Source: CAD feature listing. Evaluate the final solid. Frame: model axes, mm. A direction names the side the tool comes from. Give positions to 0.01 mm unless a question says otherwise; leave off trailing zeros. Loops run counter-clockwise (first coordinate to the right, second up) from the corner with the lowest first, then second, coordinate; pieces in that order, holes last. Notation, with made-up numbers: (26.25, 43) -> (70.25, 43) arc R9 cw to (70.25, 55) -> close; hole circle Ø9 at (15, 50.5). An arc over 180 degrees is marked (long way). Put each result on its own line as item: value.
Autodesk Inventor part; units mm, degrees
ref_plane "YZ Plane" through (0, 0, 0) normal (1, 0, 0) x (0, 1, 0)
ref_plane "XZ Plane" through (0, 0, 0) normal (0, 1, 0) x (-1, 0, 0)
ref_plane "XY Plane" through (0, 0, 0) normal (0, 0, 1) x (1, 0, 0)
sketch "Эскиз1" plane through (0, 0, 0) normal (0, 0, 1) x (1, 0, 0)
  line L0 (0, 0) -> (20, 0)
  line L1 (20, 0) -> (20, 25)
  line L2 (16, 29) -> (4, 29)
  line L3 (0, 25) -> (0, 0)
  line L4 (4, 29) -> (0, 25)
  line L5 (16, 29) -> (20, 25)
  point P0 (20, 29)
  point P1 (0, 29)
  dimension "d14" = 20
  dimension "d15" = 29
  dimension "d16" = 4
  dimension "d17" = 4
  dimension "d18" = 4
  dimension "d19" = 4
revolve "Вращение2" add sketch "Эскиз1" angle 360 about axis through (0, 0, 0) along (1, 0, 0)
sketch "Эскиз3" plane through (0, 0, 0) normal (-1, 0, 0) x (0, 0, 1)
  point P0 (0, 0)
  point P1 (0, 0)
hole "Отверстие2" at (0, 0, 0) direction (1, 0, 0) diameter 13 depth 5 tip angle 118 counterbore diameter 15 counterbore depth 2.5
properties part number "711121"
(1) Reachability of faces 1 (the cylindrical face through (9.92, 13.38, 25.73)), 2 (the cylindrical face through (1.268, -0.33, -7.493)) from +Z, -Z, +X, -X, +Y, -Y: full face, straight path, thin tool, end or side. Return the list, or none.
Calculated:
face 1: +X, -X
face 2: -X
(2) First-contact query: P1, Ø2, axis at x = 13.5, z = -18.5, coming from the +Y side; P2, Ø5, axis at x = 10, y = 9, coming from the -Z side; P3, Ø4, axis at x = 9, y = -10.5, coming from the +Z side. Flat tips, straight axial feed; report the tip coordinate or a pass-through.
Calculated:
P1: stops at y = 23.12
P2: stops at z = -28.26
P3: stops at z = 27.73
(3) Draft query along Z for faces 3 (the flat face through (0, 5, 6)), 4 (the flat face through (2.5, -3, -6)), 5 (the conical face through (0.25, -5.47, -24.65)). Return one class per face: released by +Z, released by -Z, zero draft, split by the parting line, or undercut.
Calculated:
face 3: zero draft
face 4: undercut
face 5: split by the parting line
(4) Section A-A on x = 16.75. Return loops of the section in (y, z).
Calculated:
outline: circle Ø56.5 at (0, 0)
(5) Line query: probe 1 along Y at (x, z) = (3.6, 0); probe 2 along Y at (x, z) = (3.9, 0); probe 3 along Z at (x, y) = (3.2, 0). Output: solid intervals per line, ascending. Write a range as from..to.
Calculated:
probe 1: y = -28.6..-6.5, 6.5..28.6
probe 2: y = -28.9..-6.5, 6.5..28.9
probe 3: z = -28.2..-6.5, 6.5..28.2
